```python
from build123d import *

# Parameters (mm, degrees)
SKETCH3_W          = 13
SKETCH3_H          = 25
CUT_EXTRUDE1_DEPTH = 27
FILLET1_R          = 4


with BuildPart() as part:
    # Sketch2 → Revolve1 (revolve)
    with BuildSketch(Plane(origin=(0, 0, 0), x_dir=(1, 0, 0), z_dir=(0, 1, 0))):
        with BuildLine():
            Line((0, -20), (0, 20))
            ThreePointArc((0, 20), (-20, 0), (0, -20))
        make_face()
    revolve(axis=Axis((0, 0, 20), (0, 0, -1)))

    # Sketch3 → Cut-Extrude1 (cut)
    with BuildSketch(Plane(origin=(0, 0, 0), x_dir=(1, 0, 0), z_dir=(0, 1, 0))):
        Rectangle(SKETCH3_W, SKETCH3_H)
    extrude(amount=-CUT_EXTRUDE1_DEPTH, mode=Mode.SUBTRACT)

    # Fillet1
    fillet1_edges = [part.edges().sort_by_distance(p)[0] for p in [
        (6.5, -7.097534783, -12.5),
        (6.5, -7.097534783, 12.5),
        (-6.5, -7.097534783, 12.5),
        (-6.5, -7.097534783, -12.5),
    ]]
    fillet(fillet1_edges, radius=FILLET1_R)


solid = part.part
```
Geometry check sheet. Reference: the model listing, model coordinates, mm. Coordinates: 2 decimals unless noted, no trailing zeros. Order: outer loops, then holes, each group sorted by start corner. A loop starts at its lowest first (then second) coordinate and runs counter-clockwise, first axis right, second up.
Item 1: Section check B-B (x = -10). Enter the section's corners in (y, z), plus the area to 3 significant figures.
Item 2: Section check C-C (z = -15.5). Enter the section's corners in (x, y).
Item 3: Mould release check, pull along Z, two halves, no side actions. Record for faces 1 (the flat face through (0, -8, -12.5)), 2 (the flat face through (0, 0, 0)): released by +Z, released by -Z, zero draft, split by the parting line, or undercut.
Item 4: Scan lines: line 1 along X through (y, z) = (-11, 11.5); line 2 along X through (y, z) = (-2, -0.5); line 3 along X through (y, z) = (5, -7). Record each from-to range of solid material in increasing order.
Item 5: Section check A-A (y = -14). Enter the section's corners in (x, z).
Item 6: Depth check by flat-ended pin: pin 1 (3 mm diameter, centred on x = 12, y = -8, fed in from +Z); pin 2 (6 mm diameter, centred on x = -10.5, z = -13, fed in from -Y); pin 3 (4 mm diameter, centred on y = 11, z = -12, fed in from +X). Enter the tip coordinate at first touch or a pass-through.
Item 7: Section check D-D (y = -1.5). Enter the section's corners in (x, z).
Check sheet entries:
1. outline: circle Ø34.64 at (0, 0)
1. area: 942 mm2
2. outline: circle Ø25.28 at (0, 0)
3. face 1: undercut
3. face 2: undercut
4. line 1: x = -12.11 to -5.15, 5.15 to 12.11
4. line 2: x = -19.89 to -6.5, 6.5 to 19.89
4. line 3: x = -18.06 to 18.06
5. outline: circle Ø28.57 at (0, 0); hole (-6.5, -8.5) arc R4 ccw to (-2.5, -12.5) - (2.5, -12.5) arc R4 ccw to (6.5, -8.5) - (6.5, 8.5) arc R4 ccw to (2.5, 12.5) - (-2.5, 12.5) arc R4 ccw to (-6.5, 8.5) - close
6. pin 1: stops at z = 15.26
6. pin 2: stops at y = -14.56
6. pin 3: stops at x = 14
7. outline: circle Ø39.89 at (0, 0); hole (-6.5, -8.5) arc R4 ccw to (-2.5, -12.5) - (2.5, -12.5) arc R4 ccw to (6.5, -8.5) - (6.5, 8.5) arc R4 ccw to (2.5, 12.5) - (-2.5, 12.5) arc R4 ccw to (-6.5, 8.5) - close
